```python
from build123d import *

# Parameters (mm, degrees)
F1_DEPTH = 58.42
F2_R     = 1.651
F3_DEPTH = 25.4
F4_W     = 50.8
F4_H     = 44.45
F5_DEPTH = 25.909
F6_W     = 52.07
F6_H     = 19.05
F7_DEPTH = 25.4


with BuildPart() as f1:
    # F0 (on Front) → F1 (new body)
    with BuildSketch(Plane.XZ):
        Polygon((63.5, 0), (0, 0), (0, -25.4), (-2.54, -25.4), (-2.54, -25.908), (0.508, -25.908), (0.508, -0.508), (62.992, -0.508), (62.992, -6.858), (66.04, -6.858), (66.04, -6.35), (63.5, -6.35), align=None)
    extrude(amount=-F1_DEPTH)

    # F2 (on face) → F3 (cut)
    with BuildSketch(Plane.XY):
        with Locations((2.7559, 53.6956)):
            Circle(F2_R)
        with Locations((2.7559, 4.699)):
            Circle(F2_R)
        with Locations((60.7441, 53.721)):
            Circle(F2_R)
        with Locations((60.7441, 4.7244)):
            Circle(F2_R)
    extrude(amount=-F3_DEPTH, mode=Mode.SUBTRACT)

    # F4 (on face) → F5 (cut, through all)
    with BuildSketch(Plane.XY):
        with Locations((31.75, 29.392602)):
            Rectangle(F4_W, F4_H)
    extrude(amount=-F5_DEPTH, mode=Mode.SUBTRACT)

    # F6 (on face) → F7 (cut)
    with BuildSketch(Plane(origin=(0, 0, 0), x_dir=(0, -1, 0), z_dir=(-1, 0, 0))):
        with Locations((-29.21, -12.7)):
            Rectangle(F6_W, F6_H)
    extrude(amount=-F7_DEPTH, mode=Mode.SUBTRACT)


solid = f1.part
```
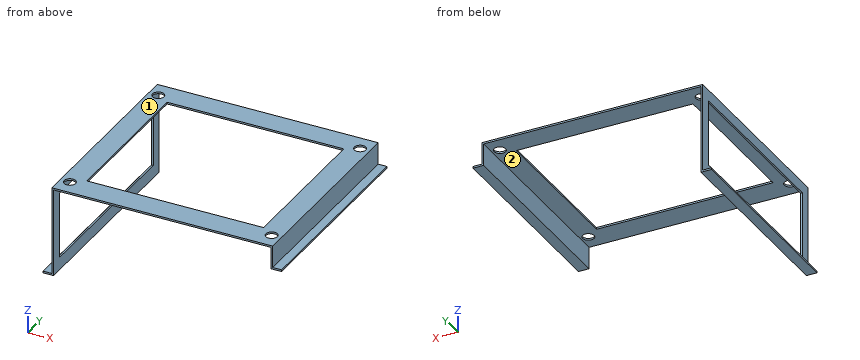
CAD build for the part. Positions are in the model's coordinates, mm. Face numbers are marked on the shaded views. A direction names the side the tool comes from. Coordinates: 2 decimals unless noted, no trailing zeros. Order: outer loops, then holes, each group sorted by start corner. A loop starts at its lowest first (then second) coordinate and runs counter-clockwise, first axis right, second up. Notation, with made-up numbers: (-10.5, -19) - (19.5, -19) arc R21 cw to (19.5, -15) - close; hole circle Ø6 at (88, 70). An arc over 180 degrees is marked (long way). Use a Markdown table: item, result. Add a question column.
(1) Flat gauge pins, fed straight in: pin 1 (1.5 mm diameter, centred on x = 65, y = 16, fed in from -Z); pin 2 (3 mm diameter, centred on y = 37, z = -3, fed in from +X); pin 3 (5 mm diameter, centred on y = 40, z = -11.5, fed in from +X); pin 4 (5 mm diameter, centred on y = 21.5, z = -2, fed in from -X). Where does each tip first touch, or does it go through?
(2) Saw through at B-B (y = 17.5). Give the cut face in (x, z) (3 decimals), then the cut area to 3 significant figures.
(3) Saw through at A-A (z = -15.75). Give the cut face in (x, y) (3 decimals), then the cut area to 3 significant figures.
(4) Drill centre lines: line 1 along X through (y, z) = (46, -3); line 2 along X through (y, z) = (2, -21.25); line 3 along Z through (x, y) = (52.5, 5). Where is each one in solid material? Low to high. Write a range as [from, to].
(5) Saw through at D-D (z = -4.5). Give the cut face in (x, y) (3 decimals), then the cut area to 3 significant figures.
(6) Which spindle directions (+Z, -Z, +X, -X, +Y, -Y) get a long thin tool onto all of the face, cutting with end or side? Do the marked faces 1 and 2. Say none if no direction does.
(7) Saw through at C-C (x = 36). Give the cut face in (y, z), then the cut area to 3 significant figures.
Solved:
| question | item | result |
|---|---|---|
| 1 | pin 1 | stops at z = -6.86 |
| 1 | pin 2 | stops at x = 63.5 |
| 1 | pin 3 | passes through |
| 1 | pin 4 | stops at x = 0 |
| 2 | outline | (-2.54, -25.908) - (0.508, -25.908) - (0.508, -22.225) - (0, -22.225) - (0, -25.4) - (-2.54, -25.4) - close; (0, -3.175) - (0.508, -3.175) - (0.508, -0.508) - (6.35, -0.508) - (6.35, 0) - (0, 0) - close; (57.15, -0.508) - (62.992, -0.508) - (62.992, -6.858) - (66.04, -6.858) - (66.04, -6.35) - (63.5, -6.35) - (63.5, 0) - (57.15, 0) - close |
| 2 | area | 15.5 mm² |
| 3 | outline | (0, 0) - (0.508, 0) - (0.508, 3.175) - (0, 3.175) - close; (0, 55.245) - (0.508, 55.245) - (0.508, 58.42) - (0, 58.42) - close |
| 3 | area | 3.23 mm² |
| 4 | line 1 | x = [0, 0.51], [62.99, 63.5] |
| 4 | line 2 | x = [0, 0.51] |
| 4 | line 3 | z = [-0.51, 0] |
| 5 | outline | (0, 0) - (0.508, 0) - (0.508, 3.175) - (0, 3.175) - close; (0, 55.245) - (0.508, 55.245) - (0.508, 58.42) - (0, 58.42) - close; (62.992, 0) - (63.5, 0) - (63.5, 58.42) - (62.992, 58.42) - close |
| 5 | area | 32.9 mm² |
| 6 | face 1 | +Z, +X, -X, +Y, -Y |
| 6 | face 2 | -Z, +Y, -Y |
| 7 | outline | (0, -0.51) - (7.17, -0.51) - (7.17, 0) - (0, 0) - close; (51.62, -0.51) - (58.42, -0.51) - (58.42, 0) - (51.62, 0) - close |
| 7 | area | 7.10 mm² |
